Autodesk Inventor part; units mm, degrees
ref_plane "FDT_MOUNT_XY" through (0, 0, 0) normal (0, 1, 0) x (-1, 0, 0)
ref_plane "FDT_MOUNT_YZ" through (0, 0, 0) normal (-1, 0, 0) x (0, 0, 1)
ref_plane "FDT_MOUNT_ZX" through (0, 0, 0) normal (0, 0, 1) x (0, 1, 0)
sketch "Sketch_4" plane through (0, 0, 0) normal (1, 0, 0) x (0, 1, 0)
  line L0 (11.3, 0) -> (16.6, 0)
  line L1 (16.6, 0) -> (16.6, -0.98)
  line L2 (16.6, -0.98) -> (15.6, -1.6)
  line L3 (15.6, -1.6) -> (16.2, -1.6)
  line L4 (16.2, -1.6) -> (16.6, -1.7865)
  line L5 (16.6, -1.7865) -> (16.6, -1.9)
  line L6 (16.6, -1.9) -> (16.4, -2.1)
  line L7 (16.4, -2.1) -> (15.6, -2.1)
  line L8 (15.6, -2.1) -> (15.6, -3.4)
  line L9 (15.6, -3.4) -> (15.3113, -3.9)
  line L10 (15.3113, -3.9) -> (11.6, -3.9)
  line L11 (11.6, -3.9) -> (11.6, -2.4)
  line L12 (11.6, -2.4) -> (0, -2.4)
  line L13 (0, -2.4) -> (0, -1.5)
  line L14 (0, -1.5) -> (-1.9935, -1.5)
  line L15 (-1.9935, -1.5) -> (-2.3, -1.1935)
  line L16 (-2.3, -1.1935) -> (-2.3, -0.8655)
  line L17 (-2.3, -0.8655) -> (-2.1, -0.75)
  line L18 (-2.1, -0.75) -> (11.3, -0.75)
  line L19 (11.3, -0.75) -> (11.3, 0)
  line L20 (11.3, 0) -> (16.6, 0)
revolve "Revolution1" add sketch "Sketch_4" angle 360 about axis through (0, 11.3, 0) along (0, 1, 0)
thread "Thread1"
sketch "Sketch_12" plane through (0, 0.3, 0) normal (0, 1, 0) x (1, 0, 0)
  arc A0 (-4, -3.6) -> (-3.6, -4) centre (-3.6, -3.6) ccw
  line L0 (-3.6, -4) -> (3.6, -4)
  arc A1 (3.6, -4) -> (4, -3.6) centre (3.6, -3.6) ccw
  line L1 (4, -3.6) -> (4, 0)
  arc A2 (4, 0) -> (-4, 0) centre (0, 0) ccw
  line L2 (-4, 0) -> (-4, -3.6)
  circle A3 centre (0, 0) radius 0.75
extrude "Extrusion1" add sketch "Sketch_12" along normal blind 11.3
sketch "Sketch_13" plane through (0, 0, 0) normal (1, 0, 0) x (0, 1, 0)
  line L0 (7, 3.5) -> (7, 6.3)
  line L1 (7, 6.3) -> (8.575, 6.3)
  line L2 (8.575, 6.3) -> (8.575, 15.5)
  arc A0 (8.875, 15.8) -> (8.575, 15.5) centre (8.875, 15.5) ccw
  line L3 (8.875, 15.8) -> (10.3347, 15.5426)
  arc A1 (10.5, 15.3456) -> (10.3347, 15.5426) centre (10.3, 15.3456) ccw
  line L4 (10.5, 15.3456) -> (10.5, 14.4)
  line L5 (10.5, 14.4) -> (9.05, 14.4)
  arc A2 (9.05, 14.4) -> (8.85, 14.2) centre (9.05, 14.2) ccw
  line L6 (8.85, 14.2) -> (8.85, 13.1)
  line L7 (8.85, 13.1) -> (9.9613, 13.1)
  line L8 (9.9613, 13.1) -> (10.25, 12.6)
  line L9 (10.25, 12.6) -> (10.25, 9.5)
  line L10 (10.25, 9.5) -> (10.9, 9.5)
  line L11 (10.9, 9.5) -> (11.1, 9.3)
  line L12 (11.1, 9.3) -> (11.1, 3.5)
  line L13 (11.1, 3.5) -> (7, 3.5)
  line L14 (7, 3.5) -> (7, 6.3)
revolve "Revolution2" add sketch "Sketch_13" angle 360 about axis through (0, 7, 3.5) along (0, 0, -1)
sketch "Sketch_14" plane through (0, 16.6, 0) normal (0, 1, 0) x (1, 0, 0)
  line L0 (-5, -6) -> (5, -6)
  line L1 (5, -6) -> (5, 6)
  line L2 (5, 6) -> (-5, 6)
  line L3 (-5, 6) -> (-5, -6)
  line L4 (-3.5, -2.0207) -> (0, -4.0415)
  line L5 (0, -4.0415) -> (3.5, -2.0207)
  line L6 (3.5, -2.0207) -> (3.5, 2.0207)
  line L7 (3.5, 2.0207) -> (0, 4.0415)
  line L8 (0, 4.0415) -> (-3.5, 2.0207)
  line L9 (-3.5, 2.0207) -> (-3.5, -2.0207)
extrude "Extrusion2" cut sketch "Sketch_14" against normal blind 4.2
sketch "Sketch_15" plane through (0, 16.6, 0) normal (0, 1, 0) x (1, 0, 0)
  line L0 (-0.3, 1.5207) -> (-0.3, -1.5207)
  arc A0 (-0.3, -1.5207) -> (0.3, -1.5207) centre (0, 0) ccw
  line L1 (0.3, -1.5207) -> (0.3, 1.5207)
  arc A1 (0.3, 1.5207) -> (-0.3, 1.5207) centre (0, 0) ccw
extrude "Extrusion3" cut sketch "Sketch_15" against normal blind 0.8
sketch "Sketch_16" plane through (0, 0, 0) normal (0, 0, 1) x (1, 0, 0)
  line L0 (-9, 35) -> (-9, -15)
  line L1 (-9, -15) -> (9, -15)
  line L2 (9, -15) -> (9, 35)
  line L3 (9, 35) -> (-9, 35)
  line L4 (-4, 31.6) -> (-4, -10)
  line L5 (-4, -10) -> (4, -10)
  line L6 (4, -10) -> (4, 31.6)
  line L7 (4, 31.6) -> (-4, 31.6)
extrude "Extrusion4" cut sketch "Sketch_16" along normal blind 15.8
sketch "Sketch_7" plane through (0, 0, 0) normal (1, 0, 0) x (0, 1, 0)
  line L0 (7, 0) -> (7, 15.8)
  line L1 (7, 15.8) -> (8.8, 15.8)
  arc A0 (8.8, 15.8) -> (8.5, 15.5) centre (8.8, 15.5) ccw
  line L2 (8.5, 15.5) -> (8.5, 6.3)
  line L3 (8.5, 6.3) -> (7.75, 6.3)
  line L4 (7.75, 6.3) -> (7.75, 0)
  line L5 (7.75, 0) -> (7, 0)
  line L6 (7, 0) -> (7, 15.8)
revolve "Revolution3" cut sketch "Sketch_7" angle 360 about axis through (0, 7, 0) along (0, 0, -1)
sketch "Sketch_17" plane through (0, 0, 15.8) normal (0, 0, 1) x (1, 0, 0)
  line L0 (-6.7662, -4.0731) -> (6.559, -4.0731)
  line L1 (6.559, -4.0731) -> (6.559, 17.5987)
  line L2 (6.559, 17.5987) -> (-6.7662, 17.5987)
  line L3 (-6.7662, 17.5987) -> (-6.7662, -4.0731)
  arc A0 (-3, 6.5) -> (3, 6.5) centre (0, 6.5) ccw
  line L4 (3, 6.5) -> (3, 7.5)
  arc A1 (3, 7.5) -> (-3, 7.5) centre (0, 7.5) ccw
  line L5 (-3, 7.5) -> (-3, 6.5)
extrude "Extrusion5" cut sketch "Sketch_17" against normal blind 1.4
ref_plane "FDT_MOUNT_XY" through (0, 0, 0) normal (0, 1, 0) x (-1, 0, 0)
ref_plane "FDT_MOUNT_YZ" through (0, 0, 0) normal (-1, 0, 0) x (0, 0, 1)
ref_plane "FDT_MOUNT_ZX" through (0, 0, 0) normal (0, 0, 1) x (0, 1, 0)
ref_plane "FDT_SCHLAUCH_XY" through (0, 7, 6.3) normal (0, 0, 1) x (1, 0, 0)
ref_plane "FDT_SCHLAUCH_YZ" through (0, 7, 6.3) normal (1, 0, 0) x (0, 1, 0)
ref_plane "FDT_SCHLAUCH_ZX" through (0, 7, 6.3) normal (0, 1, 0) x (0, 0, 1)
ref_plane "Schlauch_XY" through (0, 7, 15.8) normal (0, 0, 1) x (1, 0, 0)
ref_plane "Schlauch_YZ" through (0, 7, 15.8) normal (1, 0, 0) x (0, 1, 0)
ref_plane "Schlauch_ZX" through (0, 7, 15.8) normal (0, 1, 0) x (0, 0, 1)
ref_plane "Zylinder_XY" through (0, -2.3, 0) normal (0, 1, 0) x (1, 0, 0)
ref_plane "Zylinder_YZ" through (0, -2.3, 0) normal (1, 0, 0) x (0, 0, -1)
ref_plane "Zylinder_ZX" through (0, -2.3, 0) normal (0, 0, -1) x (0, 1, 0)
ref_plane "anbau_XY" through (0, 0, 0) normal (0, 1, 0) x (1, 0, 0)
ref_plane "anbau_YZ" through (0, 0, 0) normal (1, 0, 0) x (0, 0, -1)
ref_plane "anbau_ZX" through (0, 0, 0) normal (0, 0, -1) x (0, 1, 0)
properties part number "175043 GRLZ-M3-QS-3"
The model under review builds one solid part; all positions refer to its coordinate system, in mm. A direction names the side the tool comes from. Round coordinates to 2 decimals unless told otherwise and drop trailing zeros. Loops run counter-clockwise (first coordinate to the right, second up) from the corner with the lowest first, then second, coordinate; pieces in that order, holes last. Notation, with made-up numbers: M 74.5,39 L 129.5,39 A28 ccw 129.5,62 Z; hole C -35.75,27.5 d9. An arc over 180 degrees is marked long. Write item = value, one per line.
Item 1: Take a section at B-B on y = 2.5. Write out the cut boundary in (x, z), then the cut area to 3 significant figures.
Return value:
outline = M -4,0 A4 ccw 4,0 L 4,3.6 A0.4 ccw 3.6,4 L -3.6,4 A0.4 ccw -4,3.6 Z; hole C 0,0 d1.5
area = 55.3 mm2
Item 2: The part is to be moulded in two halves that separate along Y. For faces 1 (the flat face through (-3.5, 14, 0)), 2 (the flat face through (-1.9, 12.4, 3.2)), 3 (the cylindrical face through (-0.069, 5.427, 10.964)), say which applies: released by +Y, released by -Y, zero draft, split by the parting line, or undercut.
Return value:
face_1 = zero draft
face_2 = released by +Y
face_3 = undercut
Item 3: For line 1 (X direction, y = 7, z = 13.25) (3 decimals); line 2 (X direction, y = 7, z = 2.5); line 3 (Y direction, x = 0.75, z = -0.25), list the stretches that pass through material, from the lowest coordinate up. Write a range as [from, to].
Return value:
line_1 = [-1.85, -1.575], [1.575, 1.85]
line_2 = [-4, -0.75], [0.75, 4]
line_3 = [-2.17, 16.6]
Item 4: Machinability: for faces 4 (the cylindrical face through (0.03, 6.25, 3.11)), 5 (the cylindrical face through (0.1, 10.5, 15)), 6 (the flat face through (-3, 7, 15)), which of the approach directions +Z, -Z, +X, -X, +Y, -Y give a long, thin tool a straight path to every point of the face, cutting with its end or side? Answer none if there is none.
Return value:
face_4 = +Z
face_5 = +Z, +Y
face_6 = +Z, -X, +Y, -Y
Item 5: Insertion check: P1, Ø4.5, axis at x = 0.5, y = 6.5, coming from the +Z side; P2, Ø0.8, axis at y = 7, z = 15, coming from the -X side; P3, Ø3, axis at x = 0, y = 7, coming from the +Z side; P4, Ø0.8, axis at x = -0.5, y = 10.5, coming from the +Z side. Each pin has a flat end and moves straight along its axis. Give the tip position at first contact, or say it passes through.
Return value:
P1 = 15.8
P2 = -3
P3 = 6.3
P4 = 15.58
Item 6: Take a section at D-D on z = 11.75. Write out the cut boundary in (x, y) (3 decimals).
Return value:
outline = C 0,7 d6.5; hole C 0,7 d3.15
Item 7: Take a section at A-A on z = 4.5. Write out the cut boundary in (x, y).
Return value:
outline = M -4,6.1 A4.1 ccw 4,6.1 L 4,7.9 A4.1 ccw -4,7.9 Z; hole C 0,7 d1.5
